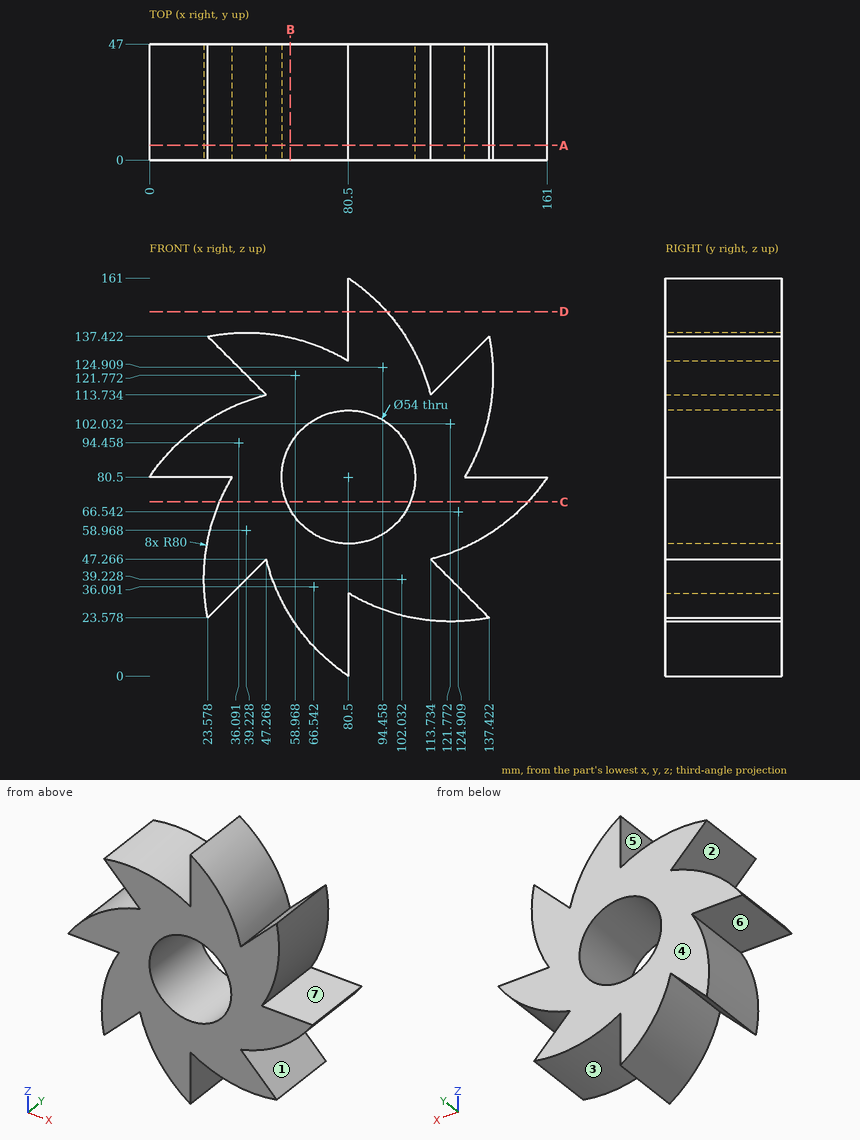
Answer from the drawing. Dimensions are ordinates in mm from the lowest x, y and z of the part. A direction names the side the tool comes from. Give positions to 0.01 mm unless a question says otherwise; leave off trailing zeros. Loops run counter-clockwise (first coordinate to the right, second up) from the corner with the lowest first, then second, coordinate; pieces in that order, holes last.
Item 1: A cutting plane is placed at D-D (z = 147.5). Give the vertices of the cut face in (x, y).
Derived:
outline: (80.5, 0) - (95.98, 0) - (95.98, 47) - (80.5, 47) - close
Item 2: A cutting plane is placed at A-A (y = 6). Give the vertices of the cut face in (x, z), then the cut area to 3 significant figures.
Derived:
outline: (0, 80.5) - (33.5, 80.5) arc R80 ccw to (23.58, 23.58) - (47.27, 47.27) arc R80 ccw to (80.5, 0) - (80.5, 33.5) arc R80 ccw to (137.42, 23.58) - (113.73, 47.27) arc R80 ccw to (161, 80.5) - (127.5, 80.5) arc R80 ccw to (137.42, 137.42) - (113.73, 113.73) arc R80 ccw to (80.5, 161) - (80.5, 127.5) arc R80 ccw to (23.58, 137.42) - (47.27, 113.73) arc R80 ccw to start; hole circle Ø54 at (80.5, 80.5)
area: 10,100 mm2
Item 3: A cutting plane is placed at C-C (z = 70.5). Give the vertices of the cut face in (x, y), then the cut area to 3 significant figures.
Derived:
outline: (28.4, 0) - (55.42, 0) - (55.42, 47) - (28.4, 47) - close; (105.58, 0) - (153.11, 0) - (153.11, 47) - (105.58, 47) - close
area: 3,500 mm2
Item 4: A cutting plane is placed at B-B (x = 57). Give the vertices of the cut face in (y, z) (1 decimal), then the cut area to 3 significant figures.
Derived:
outline: (0, 24.3) - (47, 24.3) - (47, 67.2) - (0, 67.2) - close; (0, 93.8) - (47, 93.8) - (47, 137) - (0, 137) - close
area: 4,050 mm2
Item 5: Determine the mould class of the marked faces 1, 2, 3 and 4 for opening direction X: +X half, -X half, draft (parallel to the pull), parting line (faces both ways), or undercut.
Derived:
face 1: +X half
face 2: -X half
face 3: undercut
face 4: draft
Item 6: Each of these flat-tipped pins is pushed along its axis until it touches: pin 1 Ø5 at (y, z) = (32.5, 106) entering from -X; pin 2 Ø17 at (x, y) = (152.5, 32) entering from +Z; pin 3 Ø1.5 at (x, y) = (98, 23) entering from +Z; pin 4 Ø6 at (x, z) = (48, 86) entering from -Y. Where does it stop, or does it pass through?
Derived:
pin 1: stops at x = 23.46
pin 2: stops at z = 80.5
pin 3: stops at z = 146.03
pin 4: stops at y = 0
Item 7: Find the intervals of material crossed by line 1 along X through (y, z) = (14, 131) (1 decimal); line 2 along X through (y, z) = (34.5, 67) (1 decimal); line 3 along Z through (x, y) = (86.5, 29) (1 decimal), in increasing order.
Derived:
line 1: x = 30 to 74, 80.5 to 107.3, 131 to 138.4
line 2: x = 27 to 57.1, 103.9 to 149.7
line 3: z = 30.2 to 54.2, 106.8 to 156.6
Item 8: A tool of negligible diameter and unlimited length cuts with its end or side. For the marked faces 5, 6 and 7, from which of +Z, -Z, +X, -X, +Y, -Y can it reach the whole face along a straight path? Write none if from no direction.
Derived:
face 5: +Z, +Y, -Y
face 6: -X, +Y, -Y
face 7: +X, +Y, -Y
